from build123d import *

# Parameters (mm, degrees)
F1_DEPTH  = 1
F2_W      = 5
F2_H      = 3
F3_DEPTH  = 8.5
F4_SIZE   = 2.5
F5_SIZE   = 1.5
F6_SIZE   = 0.99999
F7_R      = 0.245
F8_DEPTH  = 17
F9_W      = 5.2027019071
F9_H      = 3.5
F10_DEPTH = 1
F11_W     = 5.2027019071
F11_H     = 1.0782994613
F12_DEPTH = 6
F13_W     = 5.2027019071
F13_H     = 1.0795953252
F14_DEPTH = 6


# Not quite as in the source:
# - a fillet or chamfer is up to 0.001 mm smaller than in the source, because OpenCascade refuses the exact size


with BuildPart() as f1:
    # F0 (on Top) → F1 (new body)
    with BuildSketch(Plane.XY):
        Polygon((-12.5, -22.5), (12.5, -22.5), (12.5, -16.5), (8.5, -16.5), (8.5, -11.5), (12.5, -11.5), (12.5, 11.5), (8.5, 11.5), (8.5, 16.5), (12.5, 16.5), (12.5, 22.5), (-12.5, 22.5), (-12.5, 16.5), (-8.5, 16.5), (-8.5, 11.5), (-12.5, 11.5), (-12.5, -11.5), (-8.5, -11.5), (-8.5, -16.5), (-12.5, -16.5), align=None)
    extrude(amount=F1_DEPTH)

    # F2 (on Right) → F3 (join, symmetric)
    with BuildSketch(Plane.YZ):
        with Locations((-14, 2.5)):
            Rectangle(F2_W, F2_H)
        with Locations((14, 2.5)):
            Rectangle(F2_W, F2_H)
    extrude(amount=F3_DEPTH, both=True)

    # F4
    f4_edges = [f1.edges().sort_by_distance(p)[0] for p in [
        (12.5, -22.5, 0.5),
        (-12.5, -22.5, 0.5),
    ]]
    chamfer(f4_edges, length=F4_SIZE)

    # F5
    f5_edges = [f1.edges().sort_by_distance(p)[0] for p in [
        (12.5, 22.5, 0.5),
        (-12.5, 22.5, 0.5),
    ]]
    chamfer(f5_edges, length=F5_SIZE)

    # F6 (size 1 in the source; OpenCascade refuses exactly that, so slightly less here)
    f6_edges = [f1.edges().sort_by_distance(p)[0] for p in [
        (-11.25, -21.25, 0),
        (11.25, -21.25, 0),
    ]]
    chamfer(f6_edges, length=F6_SIZE)

    # F7 (on face) → F8 (cut)
    with BuildSketch(Plane.YZ.offset(8.5)):
        with Locations((-14, 0.5039868411)):
            Circle(F7_R)
        with Locations((14, 0.5039868411)):
            Circle(F7_R)
    extrude(amount=-F8_DEPTH, mode=Mode.SUBTRACT)

    # F9 (on face) → F10 (join)
    with BuildSketch(Plane.XY.offset(1)):
        with Locations((6.2317421885, -5.8993692152)):
            Rectangle(F9_W, F9_H)
        with Locations((-6.2317421885, -5.8993692152)):
            Rectangle(F9_W, F9_H)
        with Locations((-6.2317421885, 5.8993692152)):
            Rectangle(F9_W, F9_H)
        with Locations((6.2317421885, 5.8993692152)):
            Rectangle(F9_W, F9_H)
    extrude(amount=F10_DEPTH)

    # F11 (on face) → F12 (join)
    with BuildSketch(Plane.XY.offset(2)):
        with Locations((6.2317421885, -4.6885189459)):
            Rectangle(F11_W, F11_H)
        with Locations((-6.2317421885, -4.6885189459)):
            Rectangle(F11_W, F11_H)
    extrude(amount=F12_DEPTH)

    # F13 (on face) → F14 (join)
    with BuildSketch(Plane.XY.offset(2)):
        with Locations((6.2317421885, 7.1095715527)):
            Rectangle(F13_W, F13_H)
        with Locations((-6.2317421885, 7.1095715527)):
            Rectangle(F13_W, F13_H)
    extrude(amount=F14_DEPTH)


solid = f1.part
Could you check a few things on this model? Use its own coordinates, in mm. A direction names the side the tool comes from. Round coordinates to 2 decimals unless told otherwise and drop trailing zeros. Write each loop counter-clockwise with the first axis right and the second up, starting at its lowest first coordinate (ties: lowest second). Pieces come first, ordered by that corner, then holes. Notation, with made-up numbers: (55, 69) - (101, 69) arc R20 ccw to (101, 95) - close; hole circle Ø4 at (4.5, 75). An arc over 180 degrees is marked (long way). Use a Markdown table: item, result.
Q1. Thinking about a two-plate mould opening in Y: for faces 1 (the flat face through (0.2, 22.5, 0.5)), 2 (the flat face through (6.2, -7.649, 1.5)), 3 (the flat face through (-10.874, -20.929, 0.507)), which applies, released by +Y, released by -Y, zero draft, split by the parting line, or undercut?
Output values:
| item | result |
|---|---|
| face 1 | released by +Y |
| face 2 | undercut |
| face 3 | released by -Y |
Q2. Please list where these lines run through material, in increasing order: L1, parallel to Y at x = -5.5, z = 3.75; L2, parallel to X at y = 7.5, z = 6; L3, parallel to Y at x = 4.5, z = 4.75.
Output values:
| item | result |
|---|---|
| L1 | -16.5 to -11.5, -5.23 to -4.15, 6.57 to 7.65, 11.5 to 16.5 |
| L2 | -8.83 to -3.63, 3.63 to 8.83 |
| L3 | -5.23 to -4.15, 6.57 to 7.65 |
Q3. I want a section at B-B (x = 1). List the corners of the cut face in (y, z) for me (3 decimals).
Output values:
| item | result |
|---|---|
| outline | (-22.5, 0) - (22.5, 0) - (22.5, 1) - (16.5, 1) - (16.5, 4) - (11.5, 4) - (11.5, 1) - (-11.5, 1) - (-11.5, 4) - (-16.5, 4) - (-16.5, 1) - (-22.5, 1) - close; hole circle Ø0.49 at (-14, 0.504); hole circle Ø0.49 at (14, 0.504) |
Q4. I want a section at A-A (x = -9.25). List the corners of the cut face in (y, z) for me.
Output values:
| item | result |
|---|---|
| outline | (-22.5, 0.47) - (-21.84, 0) - (-16.5, 0) - (-16.5, 1) - (-22.5, 1) - close; (-11.5, 0) - (11.5, 0) - (11.5, 1) - (-11.5, 1) - close; (16.5, 0) - (22.5, 0) - (22.5, 1) - (16.5, 1) - close |
Q5. I want a section at C-C (y = 15.5). List the corners of the cut face in (x, z) for me.
Output values:
| item | result |
|---|---|
| outline | (-8.5, 0) - (8.5, 0) - (8.5, 4) - (-8.5, 4) - close |
Q6. For faces 4 (the flat face through (8.5, -14, 2)), 5 (the flat face through (-8.5, 14, 2)), 6 (the flat face through (8.833, 7, 4)), 7 (the flat face through (0, -16.5, 2)), which set-ups out of +Z, -Z, +X, -X, +Y, -Y let a thin tool reach every point of the face, with its end or its side?
Output values:
| item | result |
|---|---|
| face 4 | +Z, -Z, +X |
| face 5 | +Z, -Z, -X |
| face 6 | +Z, +X, +Y, -Y |
| face 7 | +Z, +X, -X, -Y |
Q7. I want a section at D-D (y = 11). List the corners of the cut face in (x, z) for me.
Output values:
| item | result |
|---|---|
| outline | (-12.5, 0) - (12.5, 0) - (12.5, 1) - (-12.5, 1) - close |
Q8. For pin 1 (4 mm diameter, centred on x = -5, z = 4.5, fed in from +Y); pin 2 (1.2 mm diameter, centred on x = 7.5, y = 5, fed in from +Z); pin 3 (1.1 mm diameter, centred on x = -10.5, z = 0.5, fed in from -Y); pin 4 (2 mm diameter, centred on y = -10, z = 2.5, fed in from +X), each with a flat end and sliding along its axis, tell me the tip position at first contact or that it passes through.
Output values:
| item | result |
|---|---|
| pin 1 | y = 16.5 |
| pin 2 | z = 2 |
| pin 3 | y = -22.25 |
| pin 4 | through |
